Geometry: see drawing. Coordinates: mm, zero at the bounding-box minimum. Round coordinates to 2 decimals unless told otherwise and drop trailing zeros. Order: outer loops, then holes, each group sorted by start corner. A loop starts at its lowest first (then second) coordinate and runs counter-clockwise, first axis right, second up. Notation, with made-up numbers: (37.25, -8.75) -> (94.25, -8.75) arc R8 cw to (94.25, 4.25) -> close; hole circle Ø11 at (16.25, 7.25). An arc over 180 degrees is marked (long way). Put each result on its own line as item: value.
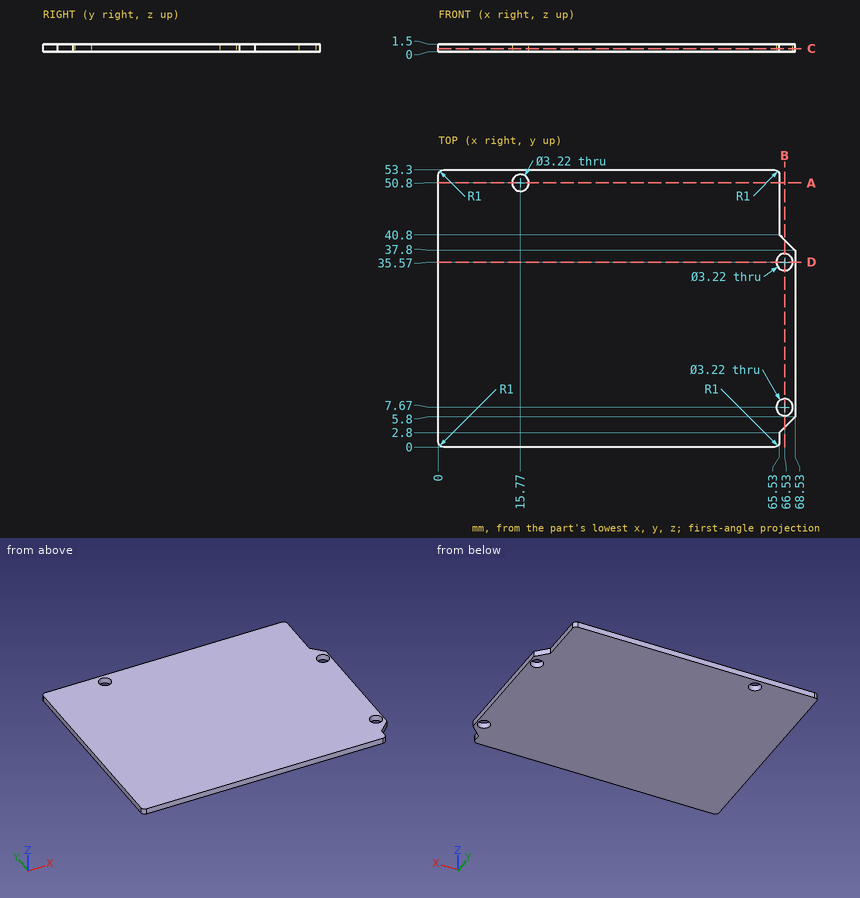
1. Cut plane D-D on y = 35.57. Return loops of the section in (x, z).
Ans:
outline: (0, 0) -> (64.92, 0) -> (64.92, 1.5) -> (0, 1.5) -> close; (68.14, 0) -> (68.53, 0) -> (68.53, 1.5) -> (68.14, 1.5) -> close
2. Cut plane C-C on z = 0.6. Return loops of the section in (x, y).
Ans:
outline: (0, 1) arc R1 ccw to (1, 0) -> (64.53, 0) arc R1 ccw to (65.53, 1) -> (65.53, 2.8) -> (68.53, 5.8) -> (68.53, 37.8) -> (65.53, 40.8) -> (65.53, 52.3) arc R1 ccw to (64.53, 53.3) -> (1, 53.3) arc R1 ccw to (0, 52.3) -> close; hole circle Ø3.22 at (15.77, 50.8); hole circle Ø3.22 at (66.53, 7.67); hole circle Ø3.22 at (66.53, 35.57)
3. Contact query for a flat-ended pin moving along its axis: P1, Ø5, axis at x = 18.5, y = 23.5, coming from the -Z side. Output: stop coordinate, or through.
Ans:
P1: z = 0
4. Material intervals for probe 1 along Y at (x, z) = (66.53, 0.6); probe 2 along Y at (x, z) = (15.77, 0.75); probe 3 along X at (y, z) = (42, 1.2), sorted ascending.
Ans:
probe 1: 3.8 to 6.06, 9.28 to 33.96, 37.18 to 39.8
probe 2: 0 to 49.19, 52.41 to 53.3
probe 3: 0 to 65.53
5. Cut plane B-B on x = 66.53. Return loops of the section in (y, z).
Ans:
outline: (3.8, 0) -> (6.06, 0) -> (6.06, 1.5) -> (3.8, 1.5) -> close; (9.28, 0) -> (33.96, 0) -> (33.96, 1.5) -> (9.28, 1.5) -> close; (37.18, 0) -> (39.8, 0) -> (39.8, 1.5) -> (37.18, 1.5) -> close
6. Cut plane A-A on y = 50.8. Return loops of the section in (x, z).
Ans:
outline: (0, 0) -> (14.16, 0) -> (14.16, 1.5) -> (0, 1.5) -> close; (17.38, 0) -> (65.53, 0) -> (65.53, 1.5) -> (17.38, 1.5) -> close
